Geometry: see drawing. Coordinates: mm, zero at the bounding-box minimum. A direction names the side the tool comes from. Give positions to 0.01 mm unless a question says otherwise; leave off trailing zeros. Loops run counter-clockwise (first coordinate to the right, second up) from the corner with the lowest first, then second, coordinate; pieces in that order, holes last. Notation, with made-up numbers: (43.25, 75.25) -> (87.25, 75.25) arc R30 cw to (87.25, 110.25) -> close; hole circle Ø7 at (62.5, 85.5). An arc over 180 degrees is marked (long way). Return JSON: item names as keys, results as strings. Group by question number.
(1) Cut plane D-D on y = 42.5. Return loops of the section in (x, z), then the cut area to 3 significant figures.
(2) Cut plane A-A on x = 19. Return loops of the section in (y, z).
(3) Draft query along Y for the marked faces 5, 6 and 7. Return one class per face: released by +Y, released by -Y, zero draft, split by the parting line, or undercut.
(4) Access query for the marked faces 1, 2, 3 and 4. Directions: +Z, -Z, +X, -X, +Y, -Y. A direction counts if a zero-diameter tool reaches every point of the face in a straight line with its end or side. Return the directions, or none.
(5) Cut plane C-C on z = 33. Return loops of the section in (x, y), then the cut area to 3 significant figures.
(6) Pin query (flat end, axial travel): pin 1 (18 mm diameter, centred on y = 22.5, z = 40, fed in from +X); pin 2 (1 mm diameter, centred on x = 27, z = 27, fed in from -Y); pin 3 (5 mm diameter, centred on x = 28.5, z = 33, fed in from +Y). Return the tip coordinate at first contact, or that it passes through.
(7) Cut plane B-B on y = 26.5. Return loops of the section in (x, z), then the cut area to 3 significant figures.
(8) Ray query, line 1 (Z direction, x = 32, y = 24); line 2 (X direction, y = 22, z = 29); line 3 (Y direction, x = 23, z = 34). Return the intervals inside material, ascending. Write a range as from..to.
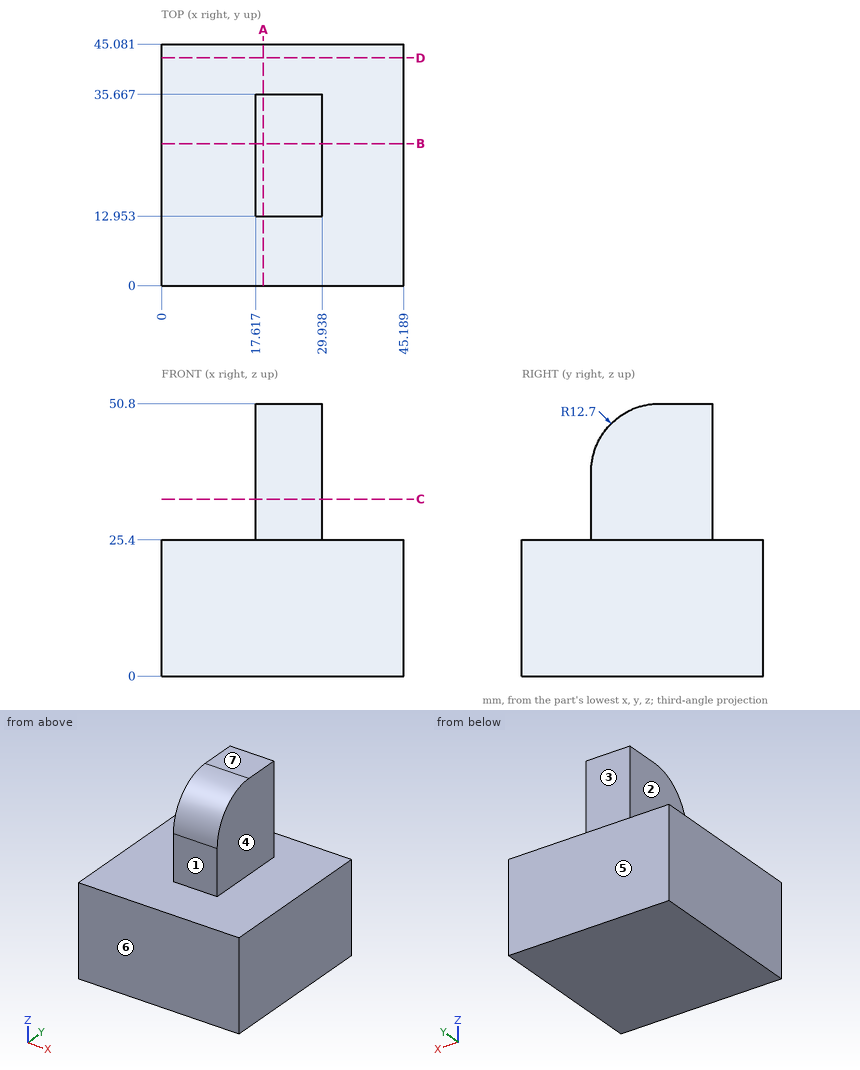
Answers:
{
 "1": {"outline": "(0, 0) -> (45.19, 0) -> (45.19, 25.4) -> (0, 25.4) -> close", "area": "1,150 mm²"},
 "2": {"outline": "(0, 0) -> (45.08, 0) -> (45.08, 25.4) -> (35.67, 25.4) -> (35.67, 50.8) -> (25.65, 50.8) arc R12.7 ccw to (12.95, 38.1) -> (12.95, 25.4) -> (0, 25.4) -> close"},
 "3": {"face 5": "released by +Y", "face 6": "released by -Y", "face 7": "zero draft"},
 "4": {"face 1": "+Z, +X, -X, -Y", "face 2": "+Z, -X, +Y, -Y", "face 3": "+Z, +X, -X, +Y", "face 4": "+Z, +X, +Y, -Y"},
 "5": {"outline": "(17.62, 12.95) -> (29.94, 12.95) -> (29.94, 35.67) -> (17.62, 35.67) -> close", "area": "280 mm²"},
 "6": {"pin 1": "x = 29.94", "pin 2": "y = 12.95", "pin 3": "y = 35.67"},
 "7": {"outline": "(0, 0) -> (45.19, 0) -> (45.19, 25.4) -> (29.94, 25.4) -> (29.94, 50.8) -> (17.62, 50.8) -> (17.62, 25.4) -> (0, 25.4) -> close", "area": "1,460 mm²"},
 "8": {"line 1": "0..25.4", "line 2": "17.62..29.94", "line 3": "12.95..35.67"}
}
